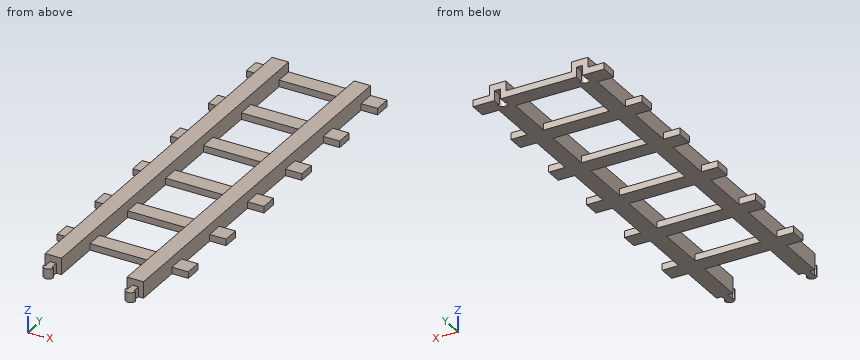
```python
from build123d import *

# Parameters (mm, degrees)
F0_W     = 6.35
F0_H     = 152.4
F1_DEPTH = 6.35
F2_W     = 50.8
F2_H     = 6.35
F3_DEPTH = 2.54
F5_DEPTH = 3.81
F7_DEPTH = 3.81


with BuildPart() as f1:
    # F0 (on Top) → F1 (new body)
    with BuildSketch(Plane.XY):
        with Locations((-15.875, 0)):
            Rectangle(F0_W, F0_H)
        with Locations((15.875, 0)):
            Rectangle(F0_W, F0_H)
    extrude(amount=F1_DEPTH)

    # F2 (on Top) → F3 (join)
    with BuildSketch(Plane.XY):
        with Locations((0, -53.975)):
            Rectangle(F2_W, F2_H)
        with Locations((0, -28.575)):
            Rectangle(F2_W, F2_H)
        with Locations((0, -3.175)):
            Rectangle(F2_W, F2_H)
        with Locations((0, 22.225)):
            Rectangle(F2_W, F2_H)
        with Locations((0, 47.625)):
            Rectangle(F2_W, F2_H)
        with Locations((0, 73.025)):
            Rectangle(F2_W, F2_H)
    extrude(amount=F3_DEPTH)

    # F4 (on face) → F5 (cut)
    with BuildSketch(Plane(origin=(0, 0, 0), x_dir=(1, 0, 0), z_dir=(0, 0, -1))):
        with BuildLine():
            Line((17.065625, -73.025), (17.78, -73.025))
            ThreePointArc((17.78, -73.025), (15.875, -71.12), (13.97, -73.025))
            Line((13.97, -73.025), (14.684375, -73.025))
            Line((14.684375, -73.025), (14.684375, -76.2))
            Line((14.684375, -76.2), (17.065625, -76.2))
            Line((17.065625, -76.2), (17.065625, -73.025))
        make_face()
        with BuildLine():
            Line((-17.78, -73.025), (-17.065625, -73.025))
            Line((-17.065625, -73.025), (-17.065625, -76.2))
            Line((-17.065625, -76.2), (-14.684375, -76.2))
            Line((-14.684375, -76.2), (-14.684375, -73.025))
            Line((-14.684375, -73.025), (-13.97, -73.025))
            ThreePointArc((-13.97, -73.025), (-15.875, -71.12), (-17.78, -73.025))
        make_face()
    extrude(amount=-F5_DEPTH, mode=Mode.SUBTRACT)

    # F6 (on face) → F7 (join)
    with BuildSketch(Plane(origin=(0, 0, 0), x_dir=(1, 0, 0), z_dir=(0, 0, -1))):
        with BuildLine():
            Line((-17.06499, 76.2), (-15.875, 76.2))
            Line((-15.875, 76.2), (-14.68501, 76.2))
            Line((-14.68501, 76.2), (-14.68501, 79.375))
            Line((-14.68501, 79.375), (-13.97127, 79.375))
            ThreePointArc((-13.97127, 79.375), (-15.875, 81.210451), (-17.77873, 79.375))
            Line((-17.77873, 79.375), (-17.06499, 79.375))
            Line((-17.06499, 79.375), (-17.06499, 76.2))
        make_face()
        with BuildLine():
            ThreePointArc((17.77873, 79.375), (15.875, 81.210451), (13.97127, 79.375))
            Line((13.97127, 79.375), (14.68501, 79.375))
            Line((14.68501, 79.375), (14.68501, 76.2))
            Line((14.68501, 76.2), (15.875, 76.2))
            Line((15.875, 76.2), (17.06499, 76.2))
            Line((17.06499, 76.2), (17.06499, 79.375))
            Line((17.06499, 79.375), (17.77873, 79.375))
        make_face()
    extrude(amount=-F7_DEPTH)


solid = f1.part
```
Geometry check sheet. Reference: the model listing, model coordinates, mm. Round coordinates to 2 decimals unless told otherwise and drop trailing zeros. Write each loop counter-clockwise with the first axis right and the second up, starting at its lowest first coordinate (ties: lowest second). Pieces come first, ordered by that corner, then holes. Notation, with made-up numbers: (36.5, -26) -> (70.5, -26) arc R20 ccw to (70.5, -9) -> close; hole circle Ø2 at (23.25, -8.5). An arc over 180 degrees is marked (long way). Put each result on its own line as item: value.
1) Depth check by flat-ended pin: P1, Ø1.3, axis at x = -21.5, z = 1.5, coming from the -Y side; P2, Ø2.5, axis at y = -77.5, z = 2.5, coming from the -X side (3 decimals); P3, Ø3, axis at y = -9, z = 3.5, coming from the -X side. Enter the tip coordinate at first touch or a pass-through.
Recorded:
P1: stops at y = -57.15
P2: stops at x = -17.065
P3: stops at x = -19.05
2) Cross-section at A-A, the plane x = 3.5. Enter the section's corners in (y, z), plus the area to 3 significant figures.
Recorded:
outline: (-57.15, 0) -> (-50.8, 0) -> (-50.8, 2.54) -> (-57.15, 2.54) -> close; (-31.75, 0) -> (-25.4, 0) -> (-25.4, 2.54) -> (-31.75, 2.54) -> close; (-6.35, 0) -> (0, 0) -> (0, 2.54) -> (-6.35, 2.54) -> close; (19.05, 0) -> (25.4, 0) -> (25.4, 2.54) -> (19.05, 2.54) -> close; (44.45, 0) -> (50.8, 0) -> (50.8, 2.54) -> (44.45, 2.54) -> close; (69.85, 0) -> (76.2, 0) -> (76.2, 2.54) -> (69.85, 2.54) -> close
area: 96.8 mm2
3) Cross-section at C-C, the plane z = 5.25. Enter the section's corners in (x, y).
Recorded:
outline: (-19.05, -76.2) -> (-12.7, -76.2) -> (-12.7, 76.2) -> (-19.05, 76.2) -> close; (12.7, -76.2) -> (19.05, -76.2) -> (19.05, 76.2) -> (12.7, 76.2) -> close
4) Thickness scan on probe 1 along Y at (x, z) = (-7, 0.5); probe 2 along X at (y, z) = (-0.5, 5.5); probe 3 along Y at (x, z) = (14.5, 5.75). Record the ranges inside material, lowest first. Write a range as from..to.
Recorded:
probe 1: y = -57.15..-50.8, -31.75..-25.4, -6.35..0, 19.05..25.4, 44.45..50.8, 69.85..76.2
probe 2: x = -19.05..-12.7, 12.7..19.05
probe 3: y = -76.2..76.2
5) Cross-section at B-B, the plane y = -41. Enter the section's corners in (x, z).
Recorded:
outline: (-19.05, 0) -> (-12.7, 0) -> (-12.7, 6.35) -> (-19.05, 6.35) -> close; (12.7, 0) -> (19.05, 0) -> (19.05, 6.35) -> (12.7, 6.35) -> close
